```python
from build123d import *

# Parameters (mm, degrees)
SKETCH1_R           = 5
BOSS_EXTRUDE2_DEPTH = 10


with BuildPart() as part:
    # Sketch1 → Boss-Extrude2 (new body)
    with BuildSketch(Plane.XY):
        with BuildLine():
            ThreePointArc((6.543934444, -2.485341424), (0, 7), (-6.543934444, -2.485341424))
            add(Edge.make_bspline(
                [(-6.543934444, -2.485341424), (-21.380303677, -6.980575662), (-40.047381701, -6.507084717), (-52.782972627, -16.427166435)],
                knots=[0.13340661, 0.13340661, 0.13340661, 0.13340661, 1, 1, 1, 1], degree=3))
            ThreePointArc((-52.782972627, -16.427166435), (-54.283149744, -21.471293509), (-50, -24.528805176))
            add(Edge.make_bspline(
                [(-50, -24.528805176), (-34.847891341, -23.200206491), (-23.436440722, -13.787418989), (-9.736135771, -9.213546422)],
                knots=[0, 0, 0, 0, 0.815262705, 0.815262705, 0.815262705, 0.815262705], degree=3))
            ThreePointArc((-9.736135771, -9.213546422), (1.368546444, -12.117530865), (12.699681517, -10.28655552))
            add(Edge.make_bspline(
                [(12.699681517, -10.28655552), (25.120949587, -15.117475017), (35.953024702, -23.297109091), (50, -24.528805176)],
                knots=[1, 1, 1, 1, 1.755800749, 1.755800749, 1.755800749, 1.755800749], degree=3))
            ThreePointArc((50, -24.528805176), (54.283149744, -21.471293509), (52.782972627, -16.427166435))
            add(Edge.make_bspline(
                [(6.543934444, -2.485341424), (21.380303677, -6.980575662), (40.047381701, -6.507084717), (52.782972627, -16.427166435)],
                knots=[0.13340661, 0.13340661, 0.13340661, 0.13340661, 1, 1, 1, 1], degree=3))
        make_face()
        Circle(SKETCH1_R, mode=Mode.SUBTRACT)
    extrude(amount=BOSS_EXTRUDE2_DEPTH)


solid = part.part
```
For this review, take the finished solid that the model builds, in its own axes (mm). Give positions to 0.01 mm unless a question says otherwise; leave off trailing zeros. Write each loop counter-clockwise with the first axis right and the second up, starting at its lowest first coordinate (ties: lowest second). Pieces come first, ordered by that corner, then holes.
Item 1: Wall thickness on probe 1 along Y at (x, z) = (0, 4.5); probe 2 along X at (y, z) = (-19, 5.25); probe 3 along X at (y, z) = (4.5, 4.75): over which ranges is each line inside the solid? List them lowest first.
Item 2: Take a section at B-B (x = 0). Give the boundary of the cut face in (y, z).
Item 3: The part is to be moulded in two halves that separate along X. For faces 1 (the face through (54.257, -21.545, 4.93)), 2 (the face through (1.21, -12.11, 4.93)), 3 (the face through (-54.308, -21.397, 4.93)), say which applies: +X half, -X half, draft (parallel to the pull), parting line (faces both ways), or undercut.
Item 4: Take a section at A-A (y = 0). Give the boundary of the cut face in (x, z).
Item 5: Insertion check: P1, Ø5, axis at x = 6.5, z = 8, coming from the -Y side. The pin has a flat end and moves straight along its axis. Give the tip position at first contact, or say it passes through.
Established:
1. probe 1: y = -12.02 to -5, 5 to 7
1. probe 2: x = -54.42 to -31.26, 31.26 to 54.42
1. probe 3: x = -5.36 to -2.18, 2.18 to 5.36
2. outline: (-12.02, 0) - (-5, 0) - (-5, 10) - (-12.02, 10) - close; (5, 0) - (7, 0) - (7, 10) - (5, 10) - close
3. face 1: +X half
3. face 2: undercut
3. face 3: -X half
4. outline: (-7, 0) - (-5, 0) - (-5, 10) - (-7, 10) - close; (5, 0) - (7, 0) - (7, 10) - (5, 10) - close
5. P1: stops at y = -12.12
